from build123d import *
from build123d.topology import SkipClean

# Parameters (mm, degrees)
BOSS_EXTRUDE1_DEPTH = 5
SKETCH2_R           = 15
BOSS_EXTRUDE2_DEPTH = 5
SKETCH3_R           = 5
CUT_EXTRUDE1_DEPTH  = 5
SKETCH4_R           = 2.5
CUT_EXTRUDE2_DEPTH  = 5
SCALE1_SCALE        = 0.6


with BuildPart() as part:
    # Sketch1 → Boss-Extrude1 (new body)
    with BuildSketch(Plane(origin=(0, 0, 0), x_dir=(1, 0, 0), z_dir=(0, 1, 0))):
        with BuildLine():
            Line((2.5, 14.790199458), (60.833333333, 4.930066486))
            ThreePointArc((60.833333333, 4.930066486), (65, 0), (60.833333333, -4.930066486))
            Line((60.833333333, -4.930066486), (2.5, -14.790199458))
            ThreePointArc((2.5, -14.790199458), (-15, 0), (2.5, 14.790199458))
        make_face()
    extrude(amount=BOSS_EXTRUDE1_DEPTH)

    # Sketch2 → Boss-Extrude2 (add)
    with SkipClean():  # the faces are left unmerged after this step: merging them gives an invalid solid
        with BuildSketch(Plane(origin=(0, 5, 0), x_dir=(1, 0, 0), z_dir=(0, 1, 0))):
            with Locations(Location((0, 0, 0), (0, 0, 80.405931773))):
                Circle(SKETCH2_R)
        extrude(amount=BOSS_EXTRUDE2_DEPTH)

    # Sketch3 → Cut-Extrude1 (cut)
    with SkipClean():  # the faces are left unmerged after this step: merging them gives an invalid solid
        with BuildSketch(Plane(origin=(0, 10, 0), x_dir=(1, 0, 0), z_dir=(0, 1, 0))):
            with Locations(Location((0, 0, 0), (0, 0, 270))):
                Circle(SKETCH3_R)
        extrude(amount=-CUT_EXTRUDE1_DEPTH, mode=Mode.SUBTRACT)

    # Sketch4 → Cut-Extrude2 (cut)
    with SkipClean():  # the faces are left unmerged after this step: merging them gives an invalid solid
        with BuildSketch(Plane(origin=(0, 5, 0), x_dir=(1, 0, 0), z_dir=(0, 1, 0))):
            with Locations(Location((50, 0, 0), (0, 0, 270))):
                Circle(SKETCH4_R)
            with Locations(Location((40, 0, 0), (0, 0, 270))):
                Circle(SKETCH4_R)
            with Locations(Location((30, 0, 0), (0, 0, 270))):
                Circle(SKETCH4_R)
        extrude(amount=-CUT_EXTRUDE2_DEPTH, mode=Mode.SUBTRACT)


with BuildPart() as part_1:
    # Scale1: scaled about (12.970813322, 3.941879124, 0)
    add(part.part.scale(SCALE1_SCALE).moved(Location((5.188325329, 1.57675165, 0))))


solid = part_1.part
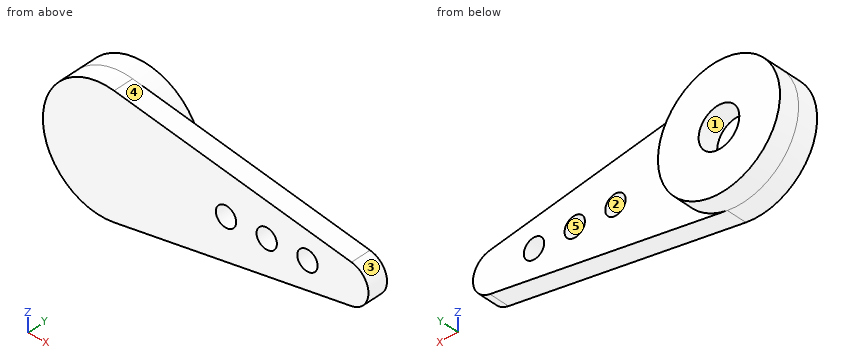
The listing builds one solid part. Answer for the finished solid, in the listing's coordinates (mm). Face numbers are marked on the shaded views. A direction names the side the tool comes from. Round coordinates to 2 decimals unless told otherwise and drop trailing zeros. Order: outer loops, then holes, each group sorted by start corner. A loop starts at its lowest first (then second) coordinate and runs counter-clockwise, first axis right, second up. Notation, with made-up numbers: M 12.5,-0.5 L 59.5,-0.5 A16 cw 59.5,6.5 Z; hole C -37,87.25 d8. An arc over 180 degrees is marked long. Answer in a Markdown table with one row per item. Add a question column.
1) Consider line 1 along X through (y, z) = (2.5, -0.5); line 2 along X through (y, z) = (6, 0); line 3 along Y through (x, z) = (36, -3.5). Determine where each line is inside the solid, lowest interval first. Write a range as from..to.
2) The part is cut by section A-A on z = 0. Determine the outline of the cut face in (x, y).
3) Determine the mould class of the marked faces 3, 4 and 5 for opening direction Z: pulls with the +Z half, pulls with the -Z half, needs draft (parallel to the pull), parting line crosses it, or undercut.
4) The part is cut by section B-B on x = 36. Determine the outline of the cut face in (y, z).
5) The part is cut by section D-D on y = 2.1. Determine the outline of the cut face in (x, z), plus the area to 3 significant figures.
6) Which of the six approach directions +Z, -Z, +X, -X, +Y, -Y give full straight-line access (tool end or side, diameter ignored) to the marked faces 1 and 2?
7) A flat-ended cylindrical pin translates along its axis: pin 1 Ø9 at (x, z) = (32, -1.5) entering from +Y. Find the tip coordinate at first contact, or state that the pin passes through.
8) The part is cut by section C-C on z = 6.25. Determine the outline of the cut face in (x, y).
Findings below:
| question | item | result |
|---|---|---|
| 1 | line 1 | x = -3.8..21.77, 24.6..27.77, 30.6..33.77, 36.6..44.15 |
| 1 | line 2 | x = -3.81..2.19, 8.19..14.19 |
| 1 | line 3 | y = 1.58..4.58 |
| 2 | outline | M -3.81,1.58 L 21.69,1.58 L 21.69,4.58 L 14.19,4.58 L 14.19,7.58 L 8.19,7.58 L 8.19,4.58 L 2.19,4.58 L 2.19,7.58 L -3.81,7.58 Z; M 24.69,1.58 L 27.69,1.58 L 27.69,4.58 L 24.69,4.58 Z; M 30.69,1.58 L 33.69,1.58 L 33.69,4.58 L 30.69,4.58 Z; M 36.69,1.58 L 44.19,1.58 L 44.19,4.58 L 36.69,4.58 Z |
| 3 | face 3 | parting line crosses it |
| 3 | face 4 | pulls with the +Z half |
| 3 | face 5 | undercut |
| 4 | outline | M 1.58,-3.92 L 4.58,-3.92 L 4.58,-1.26 L 1.58,-1.26 Z; M 1.58,1.26 L 4.58,1.26 L 4.58,3.92 L 1.58,3.92 Z |
| 5 | outline | M 6.69,-8.87 L 41.69,-2.96 A3 ccw 41.69,2.96 L 6.69,8.87 A9 ccw long Z; hole C 23.19,0 d3; hole C 29.19,0 d3; hole C 35.19,0 d3 |
| 5 | area | 558 mm² |
| 6 | face 1 | +Y |
| 6 | face 2 | +Y, -Y |
| 7 | pin 1 | stops at y = 4.58 |
| 8 | outline | M -1.29,1.58 L 22.21,1.58 L 22.21,4.58 L 11.66,4.58 L 11.66,7.58 L -1.29,7.58 Z |
